Build history of the part. All positions in model axes, mm. A direction names the side the tool comes from. Round coordinates to 2 decimals unless told otherwise and drop trailing zeros. Order: outer loops, then holes, each group sorted by start corner. A loop starts at its lowest first (then second) coordinate and runs counter-clockwise, first axis right, second up. Notation, with made-up numbers: (-24, -9.75) -> (-16, -9.75) arc R19 ccw to (-16, 7.25) -> close; hole circle Ø1 at (63.25, 59). An arc over 180 degrees is marked (long way). Use a Markdown table: item, result. Add a question column.
Item 1: Two-plate mould, pull along Y, no slides. Class faces 1 (the face through (8, 56, 0)), 2 (the face through (23.92, 81.22, 2.46)), 3 (the face through (-23.92, 28.78, 2.46)), 4 (the face through (34, 54.5, -7)): released by +Y, released by -Y, zero draft, split by the parting line, or undercut.
Item 2: 3-axis set-ups, long thin cutter, end or side, ignore diameter. For faces 5 (the face through (2.8, 59.5, 2.5)), 6 (the face through (-34, 55.5, -7)), 7 (the face through (34, 55.5, -7)): which of +Z, -Z, +X, -X, +Y, -Y reach the whole face in a straight line?
Item 3: Slice it at B-B, the plane z = -9.25. Give the cut face in (x, y), plus the area to 3 significant figures.
Item 4: Pin check, flat tips, straight feed: pin 1 (3 mm diameter, centred on x = -10, y = 35.5, fed in from -Z); pin 2 (2 mm diameter, centred on x = 28.5, z = -8, fed in from +Y); pin 3 (6 mm diameter, centred on x = 12, z = -6.5, fed in from -Y); pin 4 (9 mm diameter, centred on x = -25, y = 55, fed in from -Z). Stop position of each tip, or through.
Item 5: Slice it at A-A, the plane x = 0. Give the cut face in (y, z), plus the area to 3 significant figures.
Item 6: Slice it at D-D, the plane y = 37. Give the cut face in (x, z).
Item 7: Probe L1, parallel to X at y = 55, z = -0.75; L2, parallel to Z at x = 7.5, y = 102.5; L3, parallel to Y at x = 0, z = 2.35. List the from-to ranges inside material, lowest first.
Item 8: Slice it at C-C, the plane z = 2.75. Give the cut face in (x, y), plus the area to 3 significant figures.
from build123d import *

# Parameters (mm, degrees)
SKETCH1_R               = 5.3
BOSS_EXTRUDE1_DEPTH     = 5
BOSS_EXTRUDE2_START     = 19
SKETCH2_R               = 11
BOSS_EXTRUDE2_DEPTH     = 19
CUT_EXTRUDE1_REACH      = 120.203
SKETCH3_R               = 7.4
CUT_EXTRUDE2_REACH      = 134.834
CUT_EXTRUDE2_END_RADIUS = 7.4
SKETCH6_W               = 24
SKETCH6_H               = 1
CUT_EXTRUDE3_REACH      = 120.2
SKETCH4_R               = 1.4


with BuildPart() as part:
    # Sketch1 → Boss-Extrude1 (new body)
    with BuildSketch(Plane.XY):
        with BuildLine():
            Line((-34.788764, 60.017978), (-13.348315, 101.842697))
            ThreePointArc((-13.348315, 101.842697), (0, 110), (13.348315, 101.842697))
            Line((13.348315, 101.842697), (34.788764, 60.017978))
            ThreePointArc((34.788764, 60.017978), (36, 55), (34.788764, 49.982022))
            Line((34.788764, 49.982022), (13.348315, 8.157303))
            ThreePointArc((13.348315, 8.157303), (0, 0), (-13.348315, 8.157303))
            Line((-13.348315, 8.157303), (-34.788764, 49.982022))
            ThreePointArc((-34.788764, 49.982022), (-36, 55), (-34.788764, 60.017978))
        make_face()
        with Locations((0, 55)):
            Circle(SKETCH1_R, mode=Mode.SUBTRACT)
    extrude(amount=BOSS_EXTRUDE1_DEPTH)

    # Sketch2 → Boss-Extrude2 (add)
    with BuildSketch(Plane(origin=(0, 0, 0), x_dir=(-1, 0, 0), z_dir=(0, 0, -1)).offset(BOSS_EXTRUDE2_START)):
        with Locations((-25, 55)):
            Circle(SKETCH2_R)
        with Locations((25, 55)):
            Circle(SKETCH2_R)
    extrude(amount=-BOSS_EXTRUDE2_DEPTH)

    # Sketch3 → Cut-Extrude1 (cut, up to next)
    with BuildSketch(Plane(origin=(0, 0, -19), x_dir=(-1, 0, 0), z_dir=(0, 0, -1)), mode=Mode.PRIVATE) as cut_extrude1_sk1:
        with Locations((-25, 55)):
            Circle(SKETCH3_R)
    cut_extrude1_tool1 = extrude(cut_extrude1_sk1.sketch, amount=-CUT_EXTRUDE1_REACH, mode=Mode.PRIVATE) & part.part
    # Sketch3 → Cut-Extrude1 (cut, up to next)
    with BuildSketch(Plane(origin=(0, 0, -19), x_dir=(-1, 0, 0), z_dir=(0, 0, -1)), mode=Mode.PRIVATE) as cut_extrude1_sk2:
        with Locations((25, 55)):
            Circle(SKETCH3_R)
    cut_extrude1_tool2 = extrude(cut_extrude1_sk2.sketch, amount=-CUT_EXTRUDE1_REACH, mode=Mode.PRIVATE) & part.part
    add(cut_extrude1_tool1.solids().sort_by_distance((25, 55, -19))[0], mode=Mode.SUBTRACT)
    add(cut_extrude1_tool2.solids().sort_by_distance((-25, 55, -19))[0], mode=Mode.SUBTRACT)

    # Cut-Extrude2: up to this cylinder (the profile starts outside it)
    cut_extrude2_end = Plane(origin=(25, 55, -7), z_dir=(0, 0, -1)) * Cylinder(CUT_EXTRUDE2_END_RADIUS, 285.468, mode=Mode.PRIVATE)
    # Sketch6 → Cut-Extrude2 (cut, up to the surface)
    with BuildSketch(Plane(origin=(36, 0, 0), x_dir=(0, 0, -1), z_dir=(1, 0, 0)), mode=Mode.PRIVATE) as cut_extrude2_sk1:
        with Locations((7, 55)):
            Rectangle(SKETCH6_W, SKETCH6_H)
    cut_extrude2_tool1 = extrude(cut_extrude2_sk1.sketch, amount=-CUT_EXTRUDE2_REACH, mode=Mode.PRIVATE) - cut_extrude2_end
    cut_extrude2 = cut_extrude2_tool1.solids().sort_by_distance((36, 55, -7))[0]
    add(cut_extrude2, mode=Mode.SUBTRACT)

    # Mirror1: Cut-Extrude2 across plane
    add(cut_extrude2.mirror(Plane(origin=(0, 0, 0), x_dir=(0, 0, 1), z_dir=(1, 0, 0))), mode=Mode.SUBTRACT)

    # Sketch4 → Cut-Extrude3 (cut, up to next)
    with BuildSketch(Plane.XY.offset(5), mode=Mode.PRIVATE) as cut_extrude3_sk1:
        with Locations((-8, 55)):
            Circle(SKETCH4_R)
    cut_extrude3_tool1 = extrude(cut_extrude3_sk1.sketch, amount=-CUT_EXTRUDE3_REACH, mode=Mode.PRIVATE) & part.part
    add(cut_extrude3_tool1.solids().sort_by_distance((-8, 55, 5))[0], mode=Mode.SUBTRACT)


solid = part.part
Check sheet entries:
| question | item | result |
|---|---|---|
| 1 | face 1 | zero draft |
| 1 | face 2 | released by +Y |
| 1 | face 3 | released by -Y |
| 1 | face 4 | undercut |
| 2 | face 5 | +Z, -Z |
| 2 | face 6 | +Z, -Z, -X |
| 2 | face 7 | +Z, -Z, +X |
| 3 | outline | (-35.99, 54.5) arc R11 ccw (long way) to (-35.99, 55.5) -> (-32.38, 55.5) arc R7.4 cw (long way) to (-32.38, 54.5) -> close; (32.38, 54.5) arc R7.4 cw (long way) to (32.38, 55.5) -> (35.99, 55.5) arc R11 ccw (long way) to (35.99, 54.5) -> close |
| 3 | area | 409 mm2 |
| 4 | pin 1 | z = 0 |
| 4 | pin 2 | y = 65.71 |
| 4 | pin 3 | y = 50.42 |
| 4 | pin 4 | through |
| 5 | outline | (0, 0) -> (49.7, 0) -> (49.7, 5) -> (0, 5) -> close; (60.3, 0) -> (110, 0) -> (110, 5) -> (60.3, 5) -> close |
| 5 | area | 497 mm2 |
| 6 | outline | (-28.13, 0) -> (28.13, 0) -> (28.13, 5) -> (-28.13, 5) -> close |
| 7 | L1 | -17.6 to -14, 14 to 17.6 |
| 7 | L2 | 0 to 5 |
| 7 | L3 | 0 to 49.7, 60.3 to 110 |
| 8 | outline | (-35.99, 54.5) arc R11 ccw to (-34.79, 49.98) -> (-13.35, 8.16) arc R15 ccw to (13.35, 8.16) -> (34.79, 49.98) arc R11 ccw to (35.99, 54.5) -> (32.38, 54.5) arc R7.4 cw (long way) to (32.38, 55.5) -> (35.99, 55.5) arc R11 ccw to (34.79, 60.02) -> (13.35, 101.84) arc R15 ccw to (-13.35, 101.84) -> (-34.79, 60.02) arc R11 ccw to (-35.99, 55.5) -> (-32.38, 55.5) arc R7.4 cw (long way) to (-32.38, 54.5) -> close; hole circle Ø2.8 at (-8, 55); hole circle Ø10.6 at (0, 55) |
| 8 | area | 4,610 mm2 |
